Design review of the part built by this model. Coordinates are the model's own, in mm. A direction names the side the tool comes from. Give positions to 0.01 mm unless a question says otherwise; leave off trailing zeros. Order: outer loops, then holes, each group sorted by start corner. A loop starts at its lowest first (then second) coordinate and runs counter-clockwise, first axis right, second up.
```python
from build123d import *

# Parameters (mm, degrees)
F0_W          = 8.7122
F0_H          = 8.509
F0_W_2        = 0.6096
F0_H_2        = 12.0396
F2_R          = 4.064
F3_DEPTH      = 9.3228
F3_DEPTH_BACK = 9.3228
F4_W          = 2.794
F4_H          = 8.001
F6_W          = 0.2032
F6_H          = 0.7874
F6_W_2        = 6.1468
F8_W          = 0.508
F8_H          = 1.1684
F10_R         = 0.127
F11_SIZE      = 0.254


with BuildPart() as f1:
    # F0 (on Right) → F1 (revolve)
    with BuildSketch(Plane.YZ):
        with Locations((4.3561, 4.2545)):
            Rectangle(F0_W, F0_H)
        with Locations((4.3561, -4.2545)):
            Rectangle(F0_W, F0_H)
        with Locations((9.017, 4.2545)):
            Rectangle(F0_W_2, F0_H)
        with Locations((9.017, -4.2545)):
            Rectangle(F0_W_2, F0_H)
        with Locations((4.3561, -14.5288)):
            Rectangle(F0_W, F0_H_2)
        with Locations((4.3561, 14.5288)):
            Rectangle(F0_W, F0_H_2)
    revolve(axis=Axis((0, 0, 10.2743), (0, 0, 1)))

    # F2 (on Right) → F3 (cut, two sides)
    with BuildSketch(Plane.YZ) as f3_sk:
        Circle(F2_R)
    extrude(amount=-F3_DEPTH, mode=Mode.SUBTRACT)
    extrude(f3_sk.sketch, amount=F3_DEPTH_BACK, mode=Mode.SUBTRACT)

    # F4 (on Front) → F5 (revolve, cut)
    with BuildSketch(Plane.XZ):
        with Locations((7.9248, -4.0005)):
            Rectangle(F4_W, F4_H)
    revolve(axis=Axis((12.8778, 0, 0), (1, 0, 0)), mode=Mode.SUBTRACT)

    # F6 (on Right) → F7 (revolve, cut)
    with BuildSketch(Plane.YZ):
        Polygon((14.859, -8.509), (9.3218, -8.509), (8.7122, -8.509), (8.7122, -9.2964), (14.859, -9.2964), align=None)
        with Locations((8.6106, -8.9027)):
            Rectangle(F6_W, F6_H)
        with Locations((8.6106, 8.9027)):
            Rectangle(F6_W, F6_H)
        with Locations((11.7856, 8.9027)):
            Rectangle(F6_W_2, F6_H)
    revolve(axis=Axis((0, 0, -10.2471997961), (0, 0, -1)), mode=Mode.SUBTRACT)

    # F8 (on Right) → F9 (revolve, cut)
    with BuildSketch(Plane.YZ):
        with Locations((8.4582, -18.923)):
            Rectangle(F8_W, F8_H)
        with Locations((8.4582, 18.923)):
            Rectangle(F8_W, F8_H)
    revolve(axis=Axis((0, 0, -10.2743), (0, 0, -1)), mode=Mode.SUBTRACT)

    # F10
    f10_edges = [f1.edges().sort_by_distance(p)[0] for p in [
        (0, -8.509, -8.509),
        (0, -8.509, -9.2964),
        (0, -8.509, 8.509),
        (0, -8.509, 9.2964),
    ]]
    fillet(f10_edges, radius=F10_R)

    # F11
    f11_edges = [f1.edges().sort_by_distance(p)[0] for p in [
        (0, -8.7122, 20.5486),
        (0, -8.7122, -20.5486),
    ]]
    chamfer(f11_edges, length=F11_SIZE)


solid = f1.part
```
1. Machinability: for faces 4 (the face through (-6, 6, 19.507)), 5 (the face through (6.528, -4.3, 0.1)), 6 (the face through (0, 0, -20.549)), 7 (the face through (5.301, -6.914, -19.895)), which of the approach directions +Z, -Z, +X, -X, +Y, -Y give a long, thin tool a straight path to every point of the face, cutting with its end or side? Answer none if there is none.
Recorded:
face 4: none
face 5: +X
face 6: -Z, +X, -X, +Y, -Y
face 7: -Z
2. Take a section at B-B (z = -10.5). State the section outline as (x, y) points.
Recorded:
outline: circle Ø17.42 at (0, 0)
3. Draft analysis for pull direction Z (two halves, no side actions). For faces 1 (the face through (0, 0, 20.549)), 2 (the face through (8, 0, -8)), 3 (the face through (5.301, -6.914, 13.881)), state which applies: pulls with the +Z half, pulls with the -Z half, needs draft (parallel to the pull), parting line crosses it, or undercut.
Recorded:
face 1: pulls with the +Z half
face 2: undercut
face 3: needs draft
4. For pin 1 (5 mm diameter, centred on y = 3.5, z = 9.5, fed in from -X); pin 2 (5 mm diameter, centred on x = 2.5, z = -15.5, fed in from -Y); pin 3 (1.5 mm diameter, centred on y = -6.5, z = -8, fed in from -X), all flat-tipped, find the tip position at first contact; note any pin that passes through.
Recorded:
pin 1: stops at x = -9.24
pin 2: stops at y = -8.71
pin 3: stops at x = -7.34
5. Take a section at A-A (z = 0). State the section outline as (x, y) points.
Recorded:
outline: (-8.39, -4.06) arc R9.32 ccw to (6.53, -6.65) - (6.53, -4.06) - close; (-8.39, 4.06) - (6.53, 4.06) - (6.53, 6.65) arc R9.32 ccw to start
6. For line 1 along Z through (x, y) = (1.25, 0); line 2 along Y through (x, z) = (0.25, 0); line 3 along Y through (x, z) = (-5, 0), list the stretches that pass through material, from the lowest coordinate up.
Recorded:
line 1: z = -20.55 to -4.06, 4.06 to 20.55
line 2: y = -9.32 to -4.06, 4.06 to 9.32
line 3: y = -7.87 to -4.06, 4.06 to 7.87
